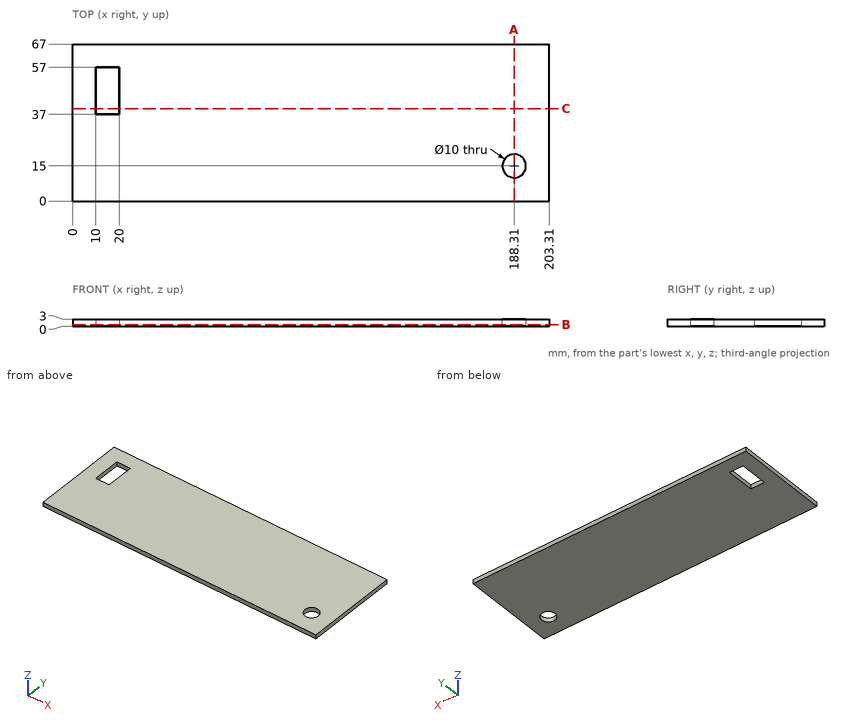
Verification items for this drawing (mm, ordinates from the low corner). Give positions to 0.01 mm unless a question says otherwise; leave off trailing zeros. Loops run counter-clockwise (first coordinate to the right, second up) from the corner with the lowest first, then second, coordinate; pieces in that order, holes last. Notation, with made-up numbers: M -20.75,57 L 30.25,57 A12 cw 30.25,61 Z; hole C 52.5,48.5 d8. An arc over 180 degrees is marked long. Answer as a JSON object with one key per item and string values. Group by question number.
Item 1: Sectioned sample at B-B on z = 0.7. Record the boundary of the cut face in (x, y), plus the area to 3 significant figures.
Item 2: Material ranges on L1, parallel to Y at x = 188.31, z = 0.65; L2, parallel to Y at x = 17, z = 1.25; L3, parallel to X at y = 16, z = 0.7, recorded low to high.
Item 3: Sectioned sample at A-A on x = 188.31. Record the boundary of the cut face in (y, z).
Item 4: Sectioned sample at C-C on y = 39.5. Record the boundary of the cut face in (x, z).
Item 5: Gauge pin test, flat end, axial feed: pin 1 (11.5 mm diameter, centred on x = 188.31, y = 15, fed in from -Z). Record the tip position at first contact, or that the pin passes through.
Findings below:
{
 "1": {"outline": "M 0,0 L 203.31,0 L 203.31,67 L 0,67 Z; hole M 10,37 L 20,37 L 20,57 L 10,57 Z; hole C 188.31,15 d10", "area": "13,300 mm2"},
 "2": {"L1": "0 to 10, 20 to 67", "L2": "0 to 37, 57 to 67", "L3": "0 to 183.41, 193.21 to 203.31"},
 "3": {"outline": "M 0,0 L 10,0 L 10,3 L 0,3 Z; M 20,0 L 67,0 L 67,3 L 20,3 Z"},
 "4": {"outline": "M 0,0 L 10,0 L 10,3 L 0,3 Z; M 20,0 L 203.31,0 L 203.31,3 L 20,3 Z"},
 "5": {"pin 1": "z = 0"}
}
